Can you work these out from the model? Positions are in its coordinate system, mm. A direction names the side the tool comes from. Round coordinates to 2 decimals unless told otherwise and drop trailing zeros. Loops run counter-clockwise (first coordinate to the right, second up) from the corner with the lowest first, then second, coordinate; pieces in that order, holes last. Notation, with made-up numbers: (-24, 81) -> (-18, 81) arc R23 cw to (-18, 102) -> close; hole circle Ø11 at (75, 31). An arc over 180 degrees is marked (long way). Answer as a JSON object with one key per item and string values.
```python
from build123d import *

# Parameters (mm, degrees)
BOSS_EXTRUDE1_DEPTH         = 76.2
FILLET1_R                   = 12.7
F_1_4_20_TAPPED_HOLE3_D     = 5.1054
F_1_4_20_TAPPED_HOLE3_DEPTH = 16.51
F_1_4_20_TAPPED_HOLE3_TIP   = 1.533816902


with BuildPart() as part:
    # Sketch1 → Boss-Extrude1 (new body)
    with BuildSketch(Plane.XY):
        Polygon((-3.386666667, 0), (31.538333333, 0), (31.538333333, 3.175), (82.338333333, 3.175), (82.338333333, 0), (117.263333333, 0), (117.263333333, 12.7), (82.338333333, 12.7), (82.338333333, 15.875), (31.538333333, 15.875), (31.538333333, 12.7), (-3.386666667, 12.7), align=None)
    extrude(amount=-BOSS_EXTRUDE1_DEPTH)

    # Fillet1
    fillet1_edges = [part.edges().sort_by_distance(p)[0] for p in [
        (117.263333333, 6.35, 0),
        (-3.386666667, 6.35, 0),
        (117.263333333, 6.35, -76.2),
        (-3.386666667, 6.35, -76.2),
    ]]
    fillet(fillet1_edges, radius=FILLET1_R)

    # 1/4-20 Tapped Hole3
    with Locations(Plane(origin=(0, 12.7, 0), x_dir=(1, 0, 0), z_dir=(0, 1, 0))):
        with Locations((104.563333333, 63.5), (104.563333333, 12.7), (9.313333333, 12.7), (9.313333333, 63.5)):
            Hole(F_1_4_20_TAPPED_HOLE3_D / 2, depth=F_1_4_20_TAPPED_HOLE3_DEPTH)
            with Locations((0, 0, -(F_1_4_20_TAPPED_HOLE3_DEPTH + F_1_4_20_TAPPED_HOLE3_TIP / 2))):  # 118° drill point
                Cone(0, F_1_4_20_TAPPED_HOLE3_D / 2, F_1_4_20_TAPPED_HOLE3_TIP, mode=Mode.SUBTRACT)


solid = part.part
```
Q1. If I drill on L1, parallel to X at y = 6, z = -63.5; L2, parallel to X at y = 2.5, z = -37.5; L3, parallel to Z at x = 103.5, y = 6.5, over which ranges is the centre line in solid material (lowest first)? Write a range as [from, to].
Determined:
{"L1": "[-3.39, 6.76], [11.87, 102.01], [107.12, 117.26]", "L2": "[-3.39, 31.54], [82.34, 117.26]", "L3": "[-76.2, -65.82], [-61.18, -15.02], [-10.38, 0]"}
Q2. I want a section at D-D, the plane y = 14.5. Write out the boundary of the cut face in (x, z), then the cut area to 3 significant figures.
Determined:
{"outline": "(31.54, -76.2) -> (82.34, -76.2) -> (82.34, 0) -> (31.54, 0) -> close", "area": "3,870 mm²"}
Q3. I want a section at B-B, the plane z = -25.5. Write out the boundary of the cut face in (x, y) (3 decimals).
Determined:
{"outline": "(-3.387, 0) -> (31.538, 0) -> (31.538, 3.175) -> (82.338, 3.175) -> (82.338, 0) -> (117.263, 0) -> (117.263, 12.7) -> (82.338, 12.7) -> (82.338, 15.875) -> (31.538, 15.875) -> (31.538, 12.7) -> (-3.387, 12.7) -> close"}
Q4. I want a section at A-A, the plane y = 7.25. Write out the boundary of the cut face in (x, z), then the cut area to 3 significant figures.
Determined:
{"outline": "(-3.39, -63.5) arc R12.7 ccw to (9.31, -76.2) -> (104.56, -76.2) arc R12.7 ccw to (117.26, -63.5) -> (117.26, -12.7) arc R12.7 ccw to (104.56, 0) -> (9.31, 0) arc R12.7 ccw to (-3.39, -12.7) -> close; hole circle Ø5.11 at (9.31, -63.5); hole circle Ø5.11 at (9.31, -12.7); hole circle Ø5.11 at (104.56, -63.5); hole circle Ø5.11 at (104.56, -12.7)", "area": "8,970 mm²"}
Q5. On a 3-axis mill with a long thin cutter (end or side, diameter ignored), from which of +Z, -Z, +X, -X, +Y, -Y can I reach the whole of each face in a straight line? I mean faces 4 (the cylindrical face through (0.235, 6.261, -3.819)), 5 (the flat face through (31.538, 2, -38)), 6 (the flat face through (31.538, 14, -38)). Say none if no direction works.
Determined:
{"face 4": "+Z, -X, +Y, -Y", "face 5": "+Z, -Z, -Y", "face 6": "+Z, -Z, -X, +Y"}
Q6. I'm going to push flat-ended pins straight in: pin 1 (1.6 mm diameter, centred on y = 14.5, z = -22, fed in from -X); pin 2 (4.5 mm diameter, centred on x = 104.56, z = -63.5, fed in from +Y) (3 decimals); pin 3 (1.5 mm diameter, centred on y = 9.5, z = -65.5, fed in from -X) (3 decimals); pin 4 (8 mm diameter, centred on x = 54.5, z = -58.5, fed in from -Y) (3 decimals). Where does each tip first touch, or does it pass through?
Determined:
{"pin 1": "x = 31.54", "pin 2": "through", "pin 3": "x = -3.325", "pin 4": "y = 3.175"}
Q7. We'd pull the mould along Z, two halves only. Please class faces 1 (the flat face through (-3.387, 6, -38)), 2 (the cylindrical face through (9.87, 6.26, -10.21)), 3 (the cylindrical face through (0.235, 6.261, -72.381)): pulls with the +Z half, pulls with the -Z half, needs draft (parallel to the pull), parting line crosses it, or undercut.
Determined:
{"face 1": "needs draft", "face 2": "undercut", "face 3": "pulls with the -Z half"}
Q8. I want a section at C-C, the plane x = 80.5. Write out the boundary of the cut face in (y, z) (3 decimals).
Determined:
{"outline": "(3.175, -76.2) -> (15.875, -76.2) -> (15.875, 0) -> (3.175, 0) -> close"}
